Read the model definition and answer for the solid it produces. Units are mm, in the model's axes. A direction names the side the tool comes from. Coordinates: 2 decimals unless noted, no trailing zeros. Order: outer loops, then holes, each group sorted by start corner. A loop starts at its lowest first (then second) coordinate and runs counter-clockwise, first axis right, second up. Notation, with made-up numbers: M 51,8 L 93,8 A9 ccw 93,24 Z; hole C -16.75,80.5 d10. An arc over 180 degrees is marked long. Use a Markdown table: item, result. Add a question column.
1) Each of these flat-tipped pins is pushed along its axis until it touches: pin 1 Ø5 at (x, y) = (-21.5, -29) entering from -Z; pin 2 Ø9 at (x, y) = (17, -22) entering from +Z; pin 3 Ø10 at (y, z) = (-18.5, 5.5) entering from +X; pin 4 Ø12 at (x, z) = (3.5, 23.5) entering from +Y. Where does it stop, or does it pass through?
2) Find section C-C on z = 32. Write down the section's boundary in (x, y).
3) Find section B-B on y = -26.5. Write down the section's boundary in (x, z).
4) For faces 1 (the face through (10.5, -37, 13)), 2 (the face through (-22, -20, 22.5)), 3 (the face through (22, -20, 22.5)), 4 (the face through (24, -20, 40.5)), 5 (the face through (-11, 0, 16)), determine the directions among +Z, -Z, +X, -X, +Y, -Y from which every point of the face is accessible in a straight line to the end or side of a thin tool.
5) The mould has two halves that part along X. Classify faces 6 (the face through (0, -20, -3)), 7 (the face through (-13.5, -20, 7)), 8 (the face through (-10.5, -14, 13)), 9 (the face through (14.93, -20.28, 21)): released by +X, released by -X, zero draft, split by the parting line, or undercut.
6) Find section D-D on x = -7. Write down the section's boundary in (y, z).
7) Find the intervals of material crossed by probe 1 along X at (y, z) = (-21, 35); probe 2 along X at (y, z) = (-22.5, 7); probe 3 along Z at (x, y) = (-23, -17), in increasing order. Write a range as [from, to].
8) Find section A-A on z = 2. Write down the section's boundary in (x, y).
from build123d import *

# Parameters (mm, degrees)
F1_DEPTH = 40
F2_R     = 5
F3_R     = 2.5
F4_DEPTH = 27


with BuildPart() as f1:
    # F0 (on Front) → F1 (new body)
    with BuildSketch(Plane.XZ):
        Polygon((10.5, 0), (0, 0), (-10.5, 0), (-10.5, 25.5), (-22, 25.5), (-22, 40.5), (-25, 40.5), (-25, 22.5), (-13.5, 22.5), (-13.5, -3), (0, -3), (13.5, -3), (13.5, 22.5), (25, 22.5), (25, 40.5), (22, 40.5), (22, 25.5), (10.5, 25.5), align=None)
    extrude(amount=F1_DEPTH)

    # F2
    f2_edges = [f1.edges().sort_by_distance(p)[0] for p in [
        (-13.5, -20, 22.5),
        (13.5, -20, 22.5),
    ]]
    fillet(f2_edges, radius=F2_R)

    # F3 (on Top) → F4 (cut)
    with BuildSketch(Plane.XY):
        with Locations((-10.423073, -31)):
            Circle(F3_R)
        with Locations((10.423073, -31)):
            Circle(F3_R)
    extrude(amount=F4_DEPTH, mode=Mode.SUBTRACT)


solid = f1.part
Check result:
| question | item | result |
|---|---|---|
| 1 | pin 1 | stops at z = 22.5 |
| 1 | pin 2 | stops at z = 25.5 |
| 1 | pin 3 | stops at x = 13.5 |
| 1 | pin 4 | passes through |
| 2 | outline | M -25,-40 L -22,-40 L -22,0 L -25,0 Z; M 22,-40 L 25,-40 L 25,0 L 22,0 Z |
| 3 | outline | M -25,22.5 L -18.5,22.5 A5 cw -13.5,17.5 L -13.5,-3 L 13.5,-3 L 13.5,17.5 A5 cw 18.5,22.5 L 25,22.5 L 25,40.5 L 22,40.5 L 22,25.5 L 10.5,25.5 L 10.5,0 L -10.5,0 L -10.5,25.5 L -22,25.5 L -22,40.5 L -25,40.5 Z |
| 4 | face 1 | +Z, +Y, -Y |
| 4 | face 2 | -Z, -X, +Y, -Y |
| 4 | face 3 | -Z, +X, +Y, -Y |
| 4 | face 4 | +Z, +X, -X, +Y, -Y |
| 4 | face 5 | +Z, -Z, +X, -X, +Y |
| 5 | face 6 | zero draft |
| 5 | face 7 | released by -X |
| 5 | face 8 | undercut |
| 5 | face 9 | released by +X |
| 6 | outline | M -40,-3 L 0,-3 L 0,0 L -40,0 Z |
| 7 | probe 1 | x = [-25, -22], [22, 25] |
| 7 | probe 2 | x = [-13.5, -10.5], [10.5, 13.5] |
| 7 | probe 3 | z = [22.5, 40.5] |
| 8 | outline | M -13.5,-40 L -10.5,-40 L -10.5,-33.5 A2.5 cw -10.5,-28.5 L -10.5,0 L -13.5,0 Z; M 10.5,-40 L 13.5,-40 L 13.5,0 L 10.5,0 L 10.5,-28.5 A2.5 cw 10.5,-33.5 Z |
